Can you work these out from the model? Positions are in its coordinate system, mm. A direction names the side the tool comes from. Give positions to 0.01 mm unless a question says otherwise; leave off trailing zeros. Loops run counter-clockwise (first coordinate to the right, second up) from the corner with the lowest first, then second, coordinate; pieces in that order, holes last. Notation, with made-up numbers: M 20,75 L 65,75 A6 ccw 65,85 Z; hole C 6,78 d1. An arc over 180 degrees is marked long. Use CSV: the item, a comma, the result in double quotes.
from build123d import *

# Parameters (mm, degrees)
F0_R     = 35
F1_DEPTH = 3
F2_R     = 5
F3_DEPTH = 5
F4_R     = 1.5
F4_R_2   = 2.5
F4_R_3   = 1.25
F5_DEPTH = 8.001
F6_W     = 70
F6_H     = 50
F7_DEPTH = 10


# Not quite as in the source:
# - a feature names something its author has since deleted; it is built from what else it names


with BuildPart() as f1:
    # F0 (on Top) → F1 (new body)
    with BuildSketch(Plane.XY):
        Circle(F0_R)
    extrude(amount=F1_DEPTH)

    # F2 (on face) → F3 (join)
    with BuildSketch(Plane(origin=(0, 0, 0), x_dir=(1, 0, 0), z_dir=(0, 0, -1))):
        Circle(F2_R)
    extrude(amount=F3_DEPTH)

    # F4 (on face) → F5 (cut, through all)
    with BuildSketch(Plane.XY.offset(3)):
        Circle(F4_R)
        with Locations((-12, 8.75)):
            Circle(F4_R_2)
        with Locations((-12, -8.75)):
            Circle(F4_R_2)
        with Locations((19, 0)):
            Circle(F4_R_3)
    extrude(amount=-F5_DEPTH, mode=Mode.SUBTRACT)

    # F6 (on Top) → F7 (intersect, symmetric)
    with BuildSketch(Plane.XY):
        Rectangle(F6_W, F6_H)
    extrude(amount=F7_DEPTH, both=True, mode=Mode.INTERSECT)


solid = f1.part
Q1. I want a section at B-B, the plane y = 0. Please give me the cut outline in (x, z), then the cut area to 4 significant figures.
Model answer:
outline,"M -35,0 L -5,0 L -5,-5 L -1.5,-5 L -1.5,3 L -35,3 Z; M 1.5,-5 L 5,-5 L 5,0 L 17.75,0 L 17.75,3 L 1.5,3 Z; M 20.25,0 L 35,0 L 35,3 L 20.25,3 Z"
area,"228.5 mm2"
Q2. For faces 1 (the cylindrical face through (-13.984, 7.229, 1.521)), 2 (the cylindrical face through (-1.08, 4.88, -2.46)), which set-ups out of +Z, -Z, +X, -X, +Y, -Y let a thin tool reach every point of the face, with its end or its side?
Model answer:
face 1,"+Z, -Z"
face 2,"-Z"
Q3. I want a section at A-A, the plane z = 1.75. Please give me the cut outline in (x, y), then the cut area to 3 significant figures.
Model answer:
outline,"M -24.49,-25 L 24.49,-25 A35 ccw 24.49,25 L -24.49,25 A35 ccw Z; hole C -12,-8.75 d5; hole C -12,8.75 d5; hole C 0,0 d3; hole C 19,0 d2.5"
area,"3,120 mm2"
Q4. I want a section at D-D, the plane x = -4. Please give me the cut outline in (y, z), then the cut area to 3 significant figures.
Model answer:
outline,"M -25,0 L -3,0 L -3,-5 L 3,-5 L 3,0 L 25,0 L 25,3 L -25,3 Z"
area,"180 mm2"
Q5. I want a section at C-C, the plane x = 19. Please give me the cut outline in (y, z), then the cut area to 4 significant figures.
Model answer:
outline,"M -25,0 L -1.25,0 L -1.25,3 L -25,3 Z; M 1.25,0 L 25,0 L 25,3 L 1.25,3 Z"
area,"142.5 mm2"
Q6. I'm going to push flat-ended pins straight in: P1, Ø4.5, axis at x = -12, y = -8.75, coming from the -Z side; P2, Ø12, axis at x = 0, y = 16.5, coming from the -Z side. Where does each tip first touch, or does it pass through?
Model answer:
P1,"through"
P2,"z = 0"
Q7. If we mould it in two halves opening along X, with no side actions, what happens to faces 3 (the cylindrical face through (35, 0, 1)), 4 (the cylindrical face through (-13.984, -10.271, 1.521)), 5 (the flat face through (-0.5, -5.2, 0))? For each: released by +X, released by -X, zero draft, split by the parting line, or undercut.
Model answer:
face 3,"released by +X"
face 4,"undercut"
face 5,"zero draft"
Q8. Please list where these lines run through material, in increasing order: L1, parallel to Y at x = -12, z = 1.45; L2, parallel to Z at x = 14, y = 10; L3, parallel to Y at x = 0, z = 0.75. Write a range as from..to.
Model answer:
L1,"-25..-11.25, -6.25..6.25, 11.25..25"
L2,"0..3"
L3,"-25..-1.5, 1.5..25"
